```python
from build123d import *

# Parameters (mm, degrees)
F0_W     = 38.1
F0_H     = 38.1
F0_W_2   = 31.75
F0_H_2   = 31.75
F1_DEPTH = 508
F2_R     = 4.7625
F3_DEPTH = 38.101
F4_R     = 4.7625
F5_DEPTH = 38.101
F6_R     = 4.7625
F7_DEPTH = 38.101


with BuildPart() as f1:
    # F0 (on Top) → F1 (new body)
    with BuildSketch(Plane.XY):
        with Locations((19.05, 19.05)):
            Rectangle(F0_W, F0_H)
        with Locations((19.05, 19.05)):
            Rectangle(F0_W_2, F0_H_2, mode=Mode.SUBTRACT)
    extrude(amount=F1_DEPTH)

    # F2 (on face) → F3 (cut, through all)
    with BuildSketch(Plane.XZ):
        with Locations((19.05, 19.05)):
            Circle(F2_R)
    extrude(amount=-F3_DEPTH, mode=Mode.SUBTRACT)

    # F4 (on face) → F5 (cut, through all)
    with BuildSketch(Plane.XZ):
        with Locations((19.05, 422.275)):
            Circle(F4_R)
    extrude(amount=-F5_DEPTH, mode=Mode.SUBTRACT)

    # F6 (on face) → F7 (cut, through all)
    with BuildSketch(Plane.XZ):
        with Locations((19.05, 469.9)):
            Circle(F6_R)
    extrude(amount=-F7_DEPTH, mode=Mode.SUBTRACT)


solid = f1.part
```
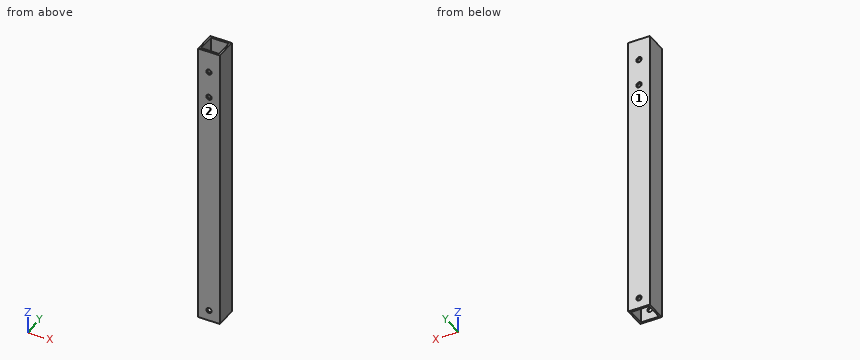
The model under review builds one solid part; all positions refer to its coordinate system, in mm. Face numbers are marked on the shaded views. Round coordinates to 2 decimals unless told otherwise and drop trailing zeros. Order: outer loops, then holes, each group sorted by start corner. A loop starts at its lowest first (then second) coordinate and runs counter-clockwise, first axis right, second up. Notation, with made-up numbers: (-20, 71.5) -> (-3, 71.5) arc R11 ccw to (-3, 89.5) -> close; hole circle Ø10 at (82, 59). An arc over 180 degrees is marked (long way). One line per item, written item: value. Start each with the question number.
Q1. Take a section at D-D (z = 274). Write out the cut boundary in (x, y) (3 decimals), and give its area (3 significant figures).
Q2. Mouldability with a two-part tool opening along Y and no side actions: class the marked faces 1 and 2 as released by +Y, released by -Y, zero draft, split by the parting line, or undercut.
Q3. Take a section at A-A (x = 9). Write out the cut boundary in (y, z) (3 decimals), and give its area (3 significant figures).
Q4. Wall thickness on line 1 (Z direction, x = 19, y = 36); line 2 (Y direction, x = 7, z = 442.5) (3 decimals): over which ranges is each line inside the solid? List them lowest first.
Q5. Clearance check with flat-ended pins moving along their axes: pin 1 Ø8.5 at (x, z) = (19.05, 422.275) entering from -Y; pin 2 Ø15 at (x, z) = (19.05, 19.05) entering from +Y. State where each tip first meets the part, or that it passes through.
Q6. Take a section at B-B (z = 19.05). Write out the cut boundary in (x, y) (1 decimal), and give its area (3 significant figures).
Reported:
1. outline: (0, 0) -> (38.1, 0) -> (38.1, 38.1) -> (0, 38.1) -> close; hole (3.175, 3.175) -> (34.925, 3.175) -> (34.925, 34.925) -> (3.175, 34.925) -> close
1. area: 444 mm2
2. face 1: released by +Y
2. face 2: released by -Y
3. outline: (0, 0) -> (3.175, 0) -> (3.175, 508) -> (0, 508) -> close; (34.925, 0) -> (38.1, 0) -> (38.1, 508) -> (34.925, 508) -> close
3. area: 3,230 mm2
4. line 1: z = 0 to 14.29, 23.81 to 417.51, 427.04 to 465.14, 474.66 to 508
4. line 2: y = 0 to 3.175, 34.925 to 38.1
5. pin 1: passes through
5. pin 2: stops at y = 38.1
6. outline: (0, 0) -> (14.3, 0) -> (14.3, 3.2) -> (3.2, 3.2) -> (3.2, 34.9) -> (14.3, 34.9) -> (14.3, 38.1) -> (0, 38.1) -> close; (23.8, 0) -> (38.1, 0) -> (38.1, 38.1) -> (23.8, 38.1) -> (23.8, 34.9) -> (34.9, 34.9) -> (34.9, 3.2) -> (23.8, 3.2) -> close
6. area: 383 mm2
